```python
from build123d import *

# Parameters (mm, degrees)
BOSS_EXTRUDE1_DEPTH     = 28.575
SKETCH2_R               = 10.3251
BOSS_EXTRUDE2_DEPTH     = 7.6962
SKETCH3_R               = 14.351
BOSS_EXTRUDE3_DEPTH     = 3.0607
SKETCH6_R               = 11.7348
CUT_EXTRUDE1_DEPTH      = 19.9771
SKETCH7_R               = 6.3373
CUT_EXTRUDE2_DEPTH      = 72.2884
CUT_EXTRUDE3_DEPTH      = 103.717779464
CUT_EXTRUDE3_DEPTH_BACK = 103.717779464
SKETCH15_W              = 20.5867
SKETCH15_H              = 9.3726
SKETCH15_H_2            = 16.0274


with BuildPart() as part:
    # Sketch1 → Boss-Extrude1 (new body)
    with BuildSketch(Plane(origin=(0, 0, 0), x_dir=(1, 0, 0), z_dir=(0, 1, 0))):
        Polygon((10.078312902, 17.45615), (-10.078312902, 17.45615), (-20.156625803, 0), (-10.078312902, -17.45615), (10.078312902, -17.45615), (20.156625803, 0), align=None)
    extrude(amount=BOSS_EXTRUDE1_DEPTH)

    # Sketch2 → Boss-Extrude2 (add)
    with BuildSketch(Plane(origin=(0, 28.575, 0), x_dir=(1, 0, 0), z_dir=(0, 1, 0))):
        with Locations(Location((0, 0, 0), (0, 0, 270))):
            Circle(SKETCH2_R)
    extrude(amount=BOSS_EXTRUDE2_DEPTH)

    # Sketch3 → Boss-Extrude3 (add)
    with BuildSketch(Plane(origin=(0, 36.2712, 0), x_dir=(1, 0, 0), z_dir=(0, 1, 0))):
        with Locations(Location((0, 0, 0), (0, 0, 270))):
            Circle(SKETCH3_R)
    extrude(amount=BOSS_EXTRUDE3_DEPTH)

    # Sketch4 → Revolve2 (revolve)
    with BuildSketch(Plane.XY, mode=Mode.PRIVATE) as revolve2_sk:
        Polygon((0, 55.3593), (9.6012, 55.3593), (10.1473, 39.3319), (0, 39.3319), align=None)
    revolve(revolve2_sk.sketch.rotate(Axis((0, 55.3593, 0), (0, -1, 0)), 180), axis=Axis((0, 55.3593, 0), (0, -1, 0)))

    # Sketch5 → Revolve3 (revolve)
    with BuildSketch(Plane.XY):
        Polygon((0, 55.3593), (10.29335, 55.3593), (9.84885, 64.7319), (0, 64.7319), align=None)
        Polygon((0, 74.1045), (0, 64.7319), (9.84885, 64.7319), (10.29335, 64.7319), (9.84885, 74.1045), align=None)
        Polygon((0, 83.4771), (0, 74.1045), (9.84885, 74.1045), (10.29335, 74.1045), (9.84885, 83.4771), align=None)
        Polygon((0, 92.8497), (0, 83.4771), (9.84885, 83.4771), (10.29335, 83.4771), (9.84885, 92.8497), align=None)
    revolve(axis=Axis((0, 55.3593, 0), (0, 1, 0)))

    # Sketch6 → Cut-Extrude1 (cut)
    with BuildSketch(Plane(origin=(0, 0, 0), x_dir=(-1, 0, 0), z_dir=(0, -1, 0))):
        with Locations(Location((0, 0, 0), (0, 0, 90))):
            Circle(SKETCH6_R)
    extrude(amount=-CUT_EXTRUDE1_DEPTH, mode=Mode.SUBTRACT)

    # Sketch7 → Cut-Extrude2 (cut)
    with BuildSketch(Plane(origin=(0, 92.8497, 0), x_dir=(1, 0, 0), z_dir=(0, 1, 0))):
        with Locations(Location((0, 0, 0), (0, 0, 180))):
            Circle(SKETCH7_R)
    extrude(amount=-CUT_EXTRUDE2_DEPTH, mode=Mode.SUBTRACT)

    # Sketch14 → Cut-Revolve1 (revolve, cut)
    with BuildSketch(Plane.XY, mode=Mode.PRIVATE) as cut_revolve1_sk:
        Polygon((6.3373, 20.5613), (0, 20.5613), (0, 19.9771), (11.7348, 19.9771), align=None)
    revolve(cut_revolve1_sk.sketch.rotate(Axis((0, 20.5613, 0), (0, -1, 0)), 180), axis=Axis((0, 20.5613, 0), (0, -1, 0)), mode=Mode.SUBTRACT)

    # Sketch15 → Cut-Extrude3 (cut, two sides: drawn at the far end of the back side and taken through both)
    with BuildSketch(Plane(origin=(15.117469352, 0, -8.728075), x_dir=(-0.4999999999999997, 0, -0.8660254037844388), z_dir=(0.8660254037844389, 0, -0.49999999999999983)).offset(-CUT_EXTRUDE3_DEPTH_BACK)):
        with Locations((0, 78.7908)):
            Rectangle(SKETCH15_W, SKETCH15_H)
        with Locations((0, 91.4908)):
            Rectangle(SKETCH15_W, SKETCH15_H_2)
    extrude(amount=CUT_EXTRUDE3_DEPTH + CUT_EXTRUDE3_DEPTH_BACK, mode=Mode.SUBTRACT)


solid = part.part
```
Model file for the job. Use its own axes, mm. A direction names the side the tool comes from. Give positions to 0.01 mm unless a question says otherwise; leave off trailing zeros. Loops run counter-clockwise (first coordinate to the right, second up) from the corner with the lowest first, then second, coordinate; pieces in that order, holes last. Notation, with made-up numbers: M 78.5,25 L 112.5,25 A9 cw 112.5,38 Z; hole C 47,-13 d7. An arc over 180 degrees is marked long. Use one line per item in the form item = value.
Item 1: Drill centre lines: L1, parallel to X at y = 13, z = 0; L2, parallel to Y at x = -5.5, z = -11 (3 decimals); L3, parallel to Z at x = 0, y = 6.5. Where is each one in solid material? Low to high.
Filled in:
L1 = -20.16 to -11.73, 11.73 to 20.16
L2 = 0 to 28.575, 36.271 to 39.332
L3 = -17.46 to -11.73, 11.73 to 17.46
Item 2: Slice it at D-D on y = 61.5. List the corners of the cut face in (x, z).
Filled in:
outline = C 0,0 d20; hole C 0,0 d12.67
Item 3: Slice it at C-C on z = 13.5. List the corners of the cut face in (x, y) (3 decimals), and give its area (3 significant figures).
Filled in:
outline = M -12.362,0 L 12.362,0 L 12.362,28.575 L -12.362,28.575 Z; M -4.868,36.271 L 4.868,36.271 L 4.868,39.332 L -4.868,39.332 Z
area = 736 mm^2
Item 4: Two-plate mould, pull along Y, no slides. Class faces 1 (the flat face through (-1, 64.732, 10)), 2 (the cylindrical face through (1.374, 47.708, -6.187)), 3 (the conical face through (5.41, 69.48, -8.49)): released by +Y, released by -Y, zero draft, split by the parting line, or undercut.
Filled in:
face_1 = undercut
face_2 = zero draft
face_3 = released by +Y
Item 5: Which spindle directions (+Z, -Z, +X, -X, +Y, -Y) get a long thin tool onto all of the face, cutting with end or side? Do faces 4 (the flat face through (9, 28.575, -8)), 5 (the cylindrical face through (-5.497, 37.78, 13.257)), 6 (the flat face through (-15.047, 14.087, -8.85)), 7 (the flat face through (15.188, 14.087, -8.606)), 8 (the cylindrical face through (-11.456, 9.849, 2.544)). Say none if no direction does.
Filled in:
face_4 = none
face_5 = +Y
face_6 = -Z, -X, +Y, -Y
face_7 = -Z, +X, +Y, -Y
face_8 = -Y
Item 6: Slice it at A-A on y = 22. List the corners of the cut face in (x, z).
Filled in:
outline = M -20.16,0 L -10.08,-17.46 L 10.08,-17.46 L 20.16,0 L 10.08,17.46 L -10.08,17.46 Z; hole C 0,0 d12.67
Item 7: Flat gauge pins, fed straight in: pin 1 Ø1 at (x, z) = (14.5, 13.5) entering from -Y; pin 2 Ø2 at (y, z) = (10, -5.5) entering from +X; pin 3 Ø8 at (y, z) = (40.5, -5) entering from -X; pin 4 Ø10.5 at (x, z) = (3, -5) entering from -Y. Where does each tip first touch, or does it go through?
Filled in:
pin_1 = through
pin_2 = 17.56
pin_3 = -14.3
pin_4 = 20.05
